Read the model definition and answer for the solid it produces. Units are mm, in the model's axes. A direction names the side the tool comes from. Give positions to 0.01 mm unless a question says otherwise; leave off trailing zeros. Write each loop counter-clockwise with the first axis right and the second up, starting at its lowest first coordinate (ties: lowest second). Pieces come first, ordered by that corner, then holes. Notation, with made-up numbers: (-28.75, -30.75) -> (4.25, -30.75) arc R4 cw to (4.25, -26.75) -> close; hole circle Ø8 at (-35, 72.5). An arc over 180 degrees is marked (long way). Answer as CSV lines item,"result". Start each with the question number.
1. A tool of negligible diameter and unlimited length cuts with its end or side. For faces 4 (the cylindrical face through (38.6, -2.44, 0.54)), 5 (the flat face through (7, -2.5, 0)), 6 (the flat face through (61.85, 0, 0)), from which of +Z, -Z, +X, -X, +Y, -Y can it reach the whole face along a straight path? Write none if from no direction.
2. The part is cut by section A-A, the plane z = 0. Determine the outline of the cut face in (x, y).
3. The part is cut by section C-C, the plane y = -5.5. Determine the outline of the cut face in (x, z), and give its area (3 significant figures).
4. The part is cut by section B-B, the plane y = 0. Determine the outline of the cut face in (x, z), and give its area (3 significant figures).
5. For a pull along Y with two mould halves and no side action, classify faces 1 (the cylindrical face through (5.9, 3.5, 0.1)), 2 (the cylindrical face through (7.888, 0.33, 7.493)), 3 (the cylindrical face through (5.45, -4.97, 1.43)) as pulls with the +Y half, pulls with the -Y half, needs draft (parallel to the pull), parting line crosses it, or undercut.
6. The part is cut by section D-D, the plane x = 52. Determine the outline of the cut face in (y, z).
7. Find the intervals of material crossed by line 1 (Y direction, x = 10, z = -0.25); line 2 (X direction, y = 4.25, z = 1.5); line 3 (X direction, y = -5.8, z = 0), in increasing order.
8. Given pin 1 (4 mm diameter, centred on x = 52, z = 2, fed in from -Y); pin 2 (6 mm diameter, centred on x = 10.5, y = 0.5, fed in from -Z); pin 3 (1.5 mm diameter, centred on x = 4.5, z = -1, fed in from +Y); pin 4 (3 mm diameter, centred on x = 46, z = 2, fed in from +Y), each flat-ended and moving along its own axis, determine where each tip first touches the part or whether it passes through.
from build123d import *

# Parameters (mm, degrees)
SKETCH1_R               = 7.5
BOSS_EXTRUDE1_DEPTH     = 16
SKETCH2_R               = 2.5
BOSS_EXTRUDE2_DEPTH     = 45.85
CUT_EXTRUDE1_DEPTH      = 12
CUT_EXTRUDE2_REACH      = 65.1
CUT_EXTRUDE2_END_RADIUS = 7.5
SKETCH4_R               = 1.5


with BuildPart() as part:
    # Sketch1 → Boss-Extrude1 (new body)
    with BuildSketch(Plane(origin=(0, 0, 0), x_dir=(0, 0, -1), z_dir=(1, 0, 0))):
        Circle(SKETCH1_R)
    extrude(amount=BOSS_EXTRUDE1_DEPTH)

    # Sketch2 → Boss-Extrude2 (add)
    with BuildSketch(Plane(origin=(16, 0, 0), x_dir=(0, 0, -1), z_dir=(1, 0, 0))):
        Circle(SKETCH2_R)
    extrude(amount=BOSS_EXTRUDE2_DEPTH)

    # Sketch3 → Cut-Extrude1 (cut)
    with BuildSketch(Plane.ZY):
        with BuildLine():
            Line((-2.449489743, -2.5), (2.449489743, -2.5))
            ThreePointArc((2.449489743, -2.5), (0, 3.5), (-2.449489743, -2.5))
        make_face()
    extrude(amount=-CUT_EXTRUDE1_DEPTH, mode=Mode.SUBTRACT)

    # Cut-Extrude2: up to this cylinder (the profile starts inside it)
    cut_extrude2_end = Plane(origin=(5, 0, 0), z_dir=(-1, 0, 0)) * Cylinder(CUT_EXTRUDE2_END_RADIUS, 146.2, mode=Mode.PRIVATE)
    # Sketch4 → Cut-Extrude2 (cut, up to the surface)
    with BuildSketch(Plane(origin=(0, -2.5, 0), x_dir=(1, 0, 0), z_dir=(0, 1, 0)), mode=Mode.PRIVATE) as cut_extrude2_sk1:
        with Locations(Location((5, 0, 0), (0, 0, 270))):
            Circle(SKETCH4_R)
    cut_extrude2_tool1 = extrude(cut_extrude2_sk1.sketch, amount=-CUT_EXTRUDE2_REACH, mode=Mode.PRIVATE) & cut_extrude2_end
    add(cut_extrude2_tool1.solids().sort_by_distance((5, -2.5, 0))[0], mode=Mode.SUBTRACT)


solid = part.part
Results found:
1,face 4,"+X"
1,face 5,"-X"
1,face 6,"+Z, -Z, +X, +Y, -Y"
2,outline,"(0, -7.5) -> (3.5, -7.5) -> (3.5, -2.5) -> (0, -2.5) -> close; (0, 3.5) -> (12, 3.5) -> (12, -2.5) -> (6.5, -2.5) -> (6.5, -7.5) -> (16, -7.5) -> (16, -2.5) -> (61.85, -2.5) -> (61.85, 2.5) -> (16, 2.5) -> (16, 7.5) -> (0, 7.5) -> close"
3,outline,"(0, -5.1) -> (16, -5.1) -> (16, 5.1) -> (0, 5.1) -> close; hole circle Ø3 at (5, 0)"
3,area,"156 mm²"
4,outline,"(0, -7.5) -> (16, -7.5) -> (16, -2.5) -> (61.85, -2.5) -> (61.85, 2.5) -> (16, 2.5) -> (16, 7.5) -> (0, 7.5) -> (0, 3.5) -> (12, 3.5) -> (12, -3.5) -> (0, -3.5) -> close"
4,area,"385 mm²"
5,face 1,"undercut"
5,face 2,"parting line crosses it"
5,face 3,"needs draft"
6,outline,"circle Ø5 at (0, 0)"
7,line 1,"y = -7.5 to -2.5, 3.49 to 7.5"
7,line 2,"x = 0 to 16"
7,line 3,"x = 0 to 3.5, 6.5 to 16"
8,pin 1,"stops at y = -2.5"
8,pin 2,"stops at z = -7.5"
8,pin 3,"stops at y = 7.5"
8,pin 4,"stops at y = 2.45"
